Here's the drawing with two shaded views (mm, measured from the low corner). I have some questions. Round coordinates to 2 decimals unless told otherwise and drop trailing zeros. Loops run counter-clockwise (first coordinate to the right, second up) from the corner with the lowest first, then second, coordinate; pieces in that order, holes last. Notation, with made-up numbers: M 81,-32 L 105,-32 A16 cw 105,-5 Z; hole C -37.75,-28.75 d8. An arc over 180 degrees is marked long. Answer as a JSON object with one key per item and string values.
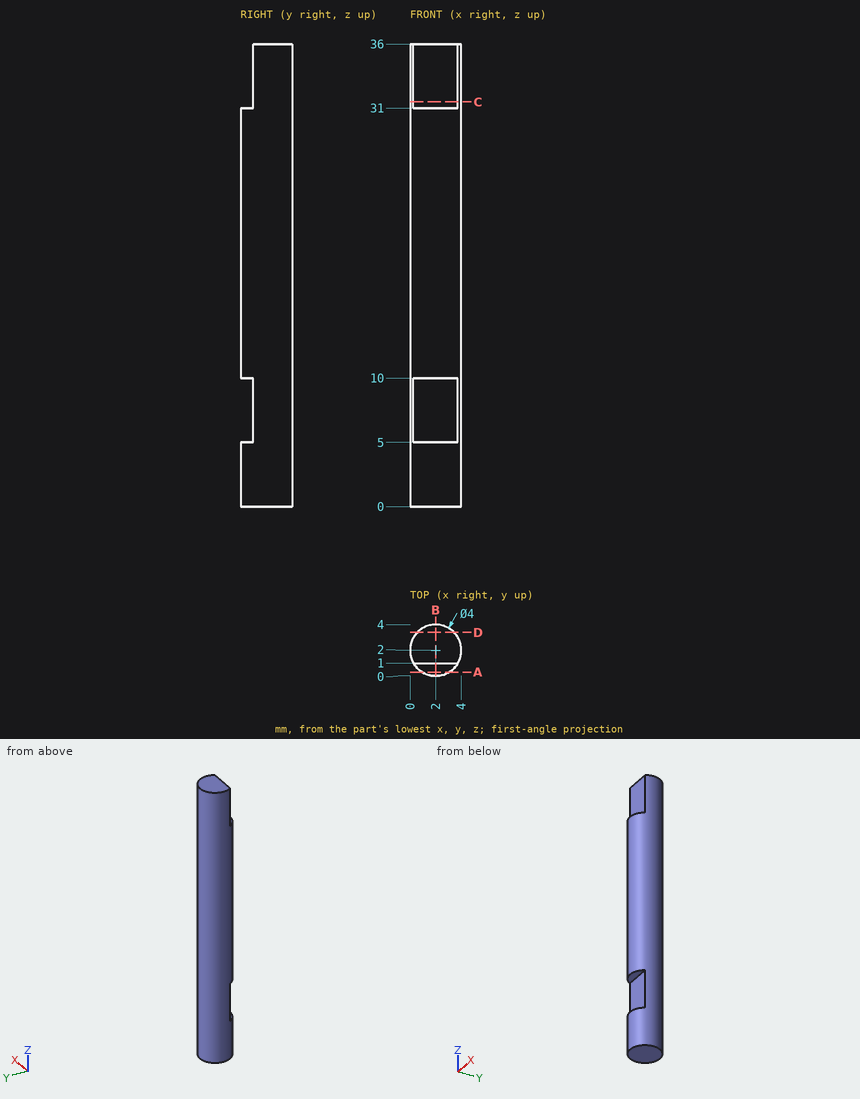
Item 1: I want a section at B-B on x = 2. List the corners of the cut face in (y, z) for me, plus the area to 3 significant figures.
Solution:
{"outline": "M 0,0 L 4,0 L 4,36 L 1,36 L 1,31 L 0,31 L 0,10 L 1,10 L 1,5 L 0,5 Z", "area": "134 mm2"}
Item 2: I want a section at C-C on z = 31.5. List the corners of the cut face in (x, y) for me.
Solution:
{"outline": "M 0.27,1 L 3.73,1 A2 ccw long Z"}
Item 3: If I drill on L1, parallel to Z at x = 0.85, y = 0.6; L2, parallel to X at y = 1.85, z = 14; L3, parallel to X at y = 3.5, z = 9.5, over which ranges is the centre line in solid material (lowest first)? Write a range as from..to.
Solution:
{"L1": "z = 0..5, 10..31", "L2": "x = 0.01..3.99", "L3": "x = 0.68..3.32"}
Item 4: I want a section at A-A on y = 0.3. List the corners of the cut face in (x, z) for me, plus the area to 3 significant figures.
Solution:
{"outline": "M 0.95,0 L 3.05,0 L 3.05,5 L 0.95,5 Z; M 0.95,10 L 3.05,10 L 3.05,31 L 0.95,31 Z", "area": "54.8 mm2"}
Item 5: I want a section at D-D on y = 3.4. List the corners of the cut face in (x, z) for me, plus the area to 3 significant figures.
Solution:
{"outline": "M 0.57,0 L 3.43,0 L 3.43,36 L 0.57,36 Z", "area": "103 mm2"}
Item 6: For P1, Ø0.5, axis at x = 1.5, y = 0.5, coming from the +Z side; P2, Ø1, axis at y = 3, z = 8.5, coming from the -X side, each with a flat end and sliding along its axis, tell me the tip position at first contact or that it passes through.
Solution:
{"P1": "stops at z = 31", "P2": "stops at x = 0.06"}
